Geometry: final body of the model. Coordinates: model frame, mm. A direction names the side the tool comes from. Give positions to 0.01 mm unless a question says otherwise; leave off trailing zeros. Order: outer loops, then holes, each group sorted by start corner. A loop starts at its lowest first (then second) coordinate and runs counter-clockwise, first axis right, second up. Notation, with made-up numbers: (22.25, 58.5) - (64.25, 58.5) arc R23 ccw to (64.25, 79.5) - close; hole circle Ø3 at (-22.5, -24). An arc over 180 degrees is marked (long way). Use one line per item in the form item = value.
from build123d import *

# Parameters (mm, degrees)
BOSS_EXTRUDE1_DEPTH = 12
SKETCH3_R           = 3
CUT_EXTRUDE1_DEPTH  = 5
BOSS_EXTRUDE2_DEPTH = 12
SKETCH5_R           = 2
CUT_EXTRUDE2_DEPTH  = 5


with BuildPart() as part:
    # Sketch1 → Boss-Extrude1 (new body)
    with BuildSketch(Plane.XY):
        Polygon((12, 0), (6, 10.392304845), (-6, 10.392304845), (-12, 0), (-6, -10.392304845), (6, -10.392304845), align=None)
    extrude(amount=BOSS_EXTRUDE1_DEPTH)

    # Sketch3 → Cut-Extrude1 (cut)
    with BuildSketch(Plane.XY.offset(12)):
        Circle(SKETCH3_R)
    extrude(amount=-CUT_EXTRUDE1_DEPTH, mode=Mode.SUBTRACT)

    # Sketch4 → Boss-Extrude2 (add)
    with BuildSketch(Plane(origin=(0, 0, 0), x_dir=(-1, 0, 0), z_dir=(0, 0, -1))):
        Polygon((12, 0), (6, 10.392304845), (-6, 10.392304845), (-12, 0), (-6, -10.392304845), (6, -10.392304845), align=None)
    extrude(amount=BOSS_EXTRUDE2_DEPTH)

    # Sketch5 → Cut-Extrude2 (cut)
    with BuildSketch(Plane(origin=(0, 0, -12), x_dir=(-1, 0, 0), z_dir=(0, 0, -1))):
        Circle(SKETCH5_R)
    extrude(amount=-CUT_EXTRUDE2_DEPTH, mode=Mode.SUBTRACT)


solid = part.part
(1) Cut plane C-C on z = 6.25. Output: boundary loops of the cut face in (x, y), plus the area to 3 significant figures.
Computed values:
outline = (-12, 0) - (-6, -10.39) - (6, -10.39) - (12, 0) - (6, 10.39) - (-6, 10.39) - close
area = 374 mm²
(2) Ray query, line 1 along Y through (x, z) = (0, 9.1); line 2 along Y through (x, z) = (0, -8.35); line 3 along X through (y, z) = (-1.5, 10.5). Return the intervals inside material, ascending.
Computed values:
line_1 = -10.39 to -3, 3 to 10.39
line_2 = -10.39 to -2, 2 to 10.39
line_3 = -11.13 to -2.6, 2.6 to 11.13
(3) Cut plane D-D on y = 0.75. Output: boundary loops of the cut face in (x, z), plus the area to 3 significant figures.
Computed values:
outline = (-11.57, -12) - (-1.85, -12) - (-1.85, -7) - (1.85, -7) - (1.85, -12) - (11.57, -12) - (11.57, 12) - (2.9, 12) - (2.9, 7) - (-2.9, 7) - (-2.9, 12) - (-11.57, 12) - close
area = 508 mm²
(4) Contact query for flat-ended pins moving along their axis: pin 1 Ø4 at (y, z) = (2.5, 9) entering from -X; pin 2 Ø1.5 at (y, z) = (-5, 9) entering from -X; pin 3 Ø3.5 at (x, y) = (0, 0) entering from +Z. Output: stop coordinate, or through.
Computed values:
pin_1 = -11.71
pin_2 = -9.55
pin_3 = 7
(5) Reachability of faces 1 (the face through (0, -2, -10)), 2 (the face through (0, -10.392, 0)), 3 (the face through (0, 0, 7)) from +Z, -Z, +X, -X, +Y, -Y: full face, straight path, thin tool, end or side. Return the list, or none.
Computed values:
face_1 = -Z
face_2 = +Z, -Z, +X, -X, -Y
face_3 = +Z
(6) Cut plane B-B on x = 0. Output: boundary loops of the cut face in (y, z), plus the area to 3 significant figures.
Computed values:
outline = (-10.39, -12) - (-2, -12) - (-2, -7) - (2, -7) - (2, -12) - (10.39, -12) - (10.39, 12) - (3, 12) - (3, 7) - (-3, 7) - (-3, 12) - (-10.39, 12) - close
area = 449 mm²
(7) Cut plane A-A on z = -7.75. Output: boundary loops of the cut face in (x, y), plus the area to 3 significant figures.
Computed values:
outline = (-12, 0) - (-6, -10.39) - (6, -10.39) - (12, 0) - (6, 10.39) - (-6, 10.39) - close; hole circle Ø4 at (0, 0)
area = 362 mm²
